Check sheet for the modelled part. Datum: model origin and axes. Units: mm. Face numbers are marked on the shaded views. Give positions to 0.01 mm unless a question says otherwise; leave off trailing zeros. Loops run counter-clockwise (first coordinate to the right, second up) from the corner with the lowest first, then second, coordinate; pieces in that order, holes last. Notation, with made-up numbers: M 58.25,88 L 92.25,88 A20 cw 92.25,108 Z; hole C 8,-24 d1. An arc over 180 degrees is marked long. Use one line per item in the form item = value.
from build123d import *

# Parameters (mm, degrees)
CYLINDER014_R     = 1.4
CYLINDER014_DEPTH = 4
CYLINDER015_R     = 3.5
CYLINDER015_DEPTH = 4


with BuildPart() as cylinder014:
    # Cylinder014 → Cylinder014 (new body)
    with BuildSketch(Plane.XY):
        Circle(CYLINDER014_R)
    extrude(amount=CYLINDER014_DEPTH)


with BuildPart() as m2p5_spacer:
    # Cylinder015 → Cylinder015 (new body)
    with BuildSketch(Plane.XY):
        Circle(CYLINDER015_R)
    extrude(amount=CYLINDER015_DEPTH)

    # Cut011: cut Cylinder014
    add(cylinder014.part, mode=Mode.SUBTRACT)


solid = m2p5_spacer.part
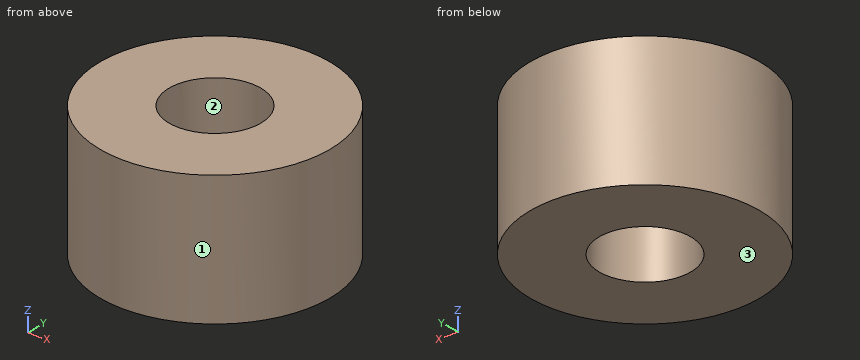
1) Section check A-A (y = 0). Record the cut outline in (x, z), then the cut area to 3 significant figures.
Evaluation:
outline = M -3.5,0 L -1.4,0 L -1.4,4 L -3.5,4 Z; M 1.4,0 L 3.5,0 L 3.5,4 L 1.4,4 Z
area = 16.8 mm^2
2) Scan lines: line 1 (Y direction, x = 0, z = 2.75); line 2 (X direction, y = -0.25, z = 2.5); line 3 (X direction, y = 1, z = 2.85). Record each from-to range of solid material in increasing order.
Evaluation:
line_1 = -3.5 to -1.4, 1.4 to 3.5
line_2 = -3.49 to -1.38, 1.38 to 3.49
line_3 = -3.35 to -0.98, 0.98 to 3.35
3) Depth check by flat-ended pin: pin 1 Ø3.5 at (x, y) = (0, 0) entering from +Z. Enter the tip coordinate at first touch or a pass-through.
Evaluation:
pin_1 = 4
4) Section check D-D (y = 2.25). Record the cut outline in (x, z).
Evaluation:
outline = M -2.68,0 L 2.68,0 L 2.68,4 L -2.68,4 Z
5) Release check for a two-part mould opening along X. For the marked faces 1, 2 and 3 record: pulls with the +X half, pulls with the -X half, needs draft (parallel to the pull), parting line crosses it, or undercut.
Evaluation:
face_1 = parting line crosses it
face_2 = undercut
face_3 = needs draft
6) Section check C-C (z = 2.4). Record the cut outline in (x, y).
Evaluation:
outline = C 0,0 d7; hole C 0,0 d2.8
